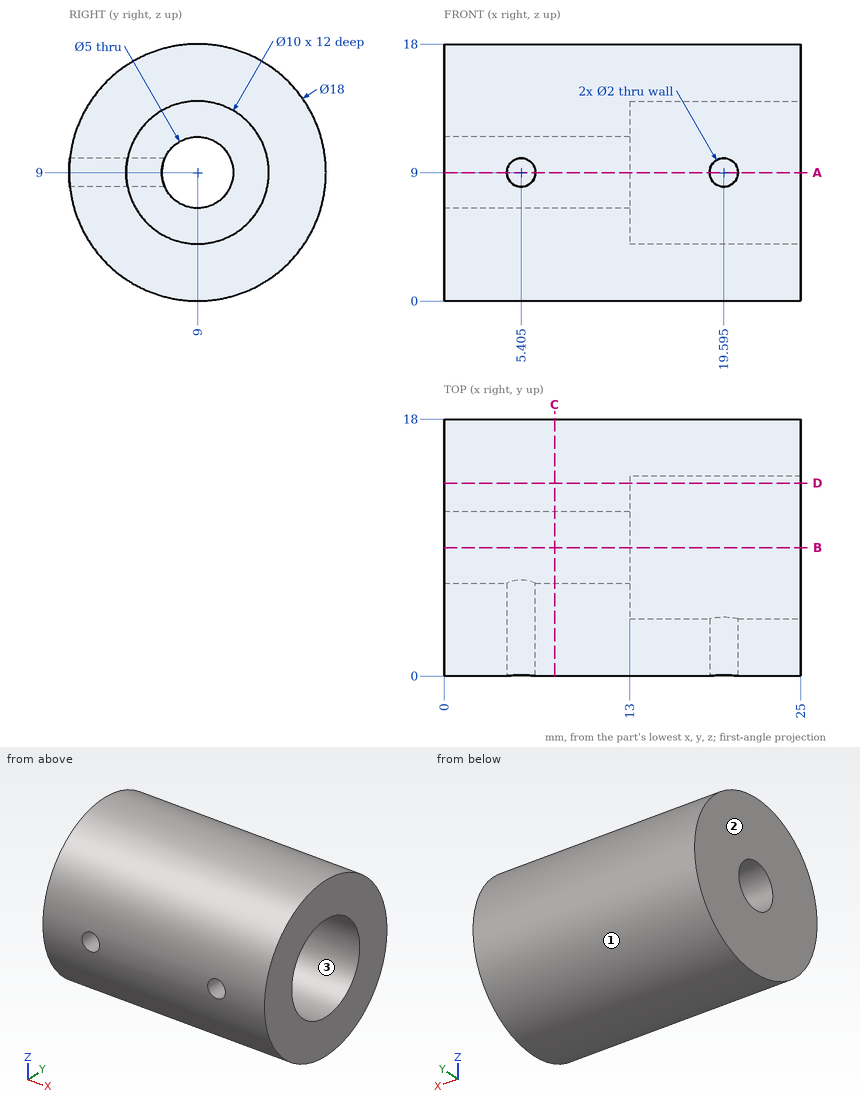
Design review of the part shown in the three views and the two pictorial views. Dimensions are in mm from the part's minimum x, y and z. Coordinates: 2 decimals unless noted, no trailing zeros. Write each loop counter-clockwise with the first axis right and the second up, starting at its lowest first coordinate (ties: lowest second). Pieces come first, ordered by that corner, then holes.
1) We need section A-A on z = 9. State the section outline as (x, y) points (1 decimal).
2) Clearance check with flat-ended pins moving along their axes: pin 1 Ø2 at (x, z) = (6.5, 14.5) entering from -Y (1 decimal); pin 2 Ø1.5 at (x, z) = (19.5, 7) entering from +Y; pin 3 Ø4 at (x, y) = (17.5, 13) entering from +Z (1 decimal). State where each tip first meets the part, or that it passes through.
3) We need section D-D on y = 13.5. State the section outline as (x, z) points (1 decimal), then the cut area to 3 significant figures.
4) We need section B-B on y = 9. State the section outline as (x, z) points.
5) We need section C-C on x = 7.75. State the section outline as (y, z) points.
6) The part is to be moulded in two halves that separate along Z. For the marked faces 1, 2 and 3, say which applies: pulls with the +Z half, pulls with the -Z half, needs draft (parallel to the pull), parting line crosses it, or undercut.
7) To check wall thickness, follow probe 1 along Z at (x, y) = (16.5, 12.25); probe 2 along Z at (x, y) = (22.5, 9); probe 3 along Y at (x, z) = (3.75, 7.5) (1 decimal). State the ranges of each line that lie inside material, in increasing order.
Answer list:
1. outline: (0, 0) - (4.4, 0) - (4.4, 6.5) - (0, 6.5) - close; (0, 11.5) - (13, 11.5) - (13, 14) - (25, 14) - (25, 18) - (0, 18) - close; (6.4, 0) - (18.6, 0) - (18.6, 4) - (13, 4) - (13, 6.5) - (6.4, 6.5) - close; (20.6, 0) - (25, 0) - (25, 4) - (20.6, 4) - close
2. pin 1: stops at y = 1.2
2. pin 2: stops at y = 17.91
2. pin 3: stops at z = 17.8
3. outline: (0, 1.2) - (25, 1.2) - (25, 6.8) - (13, 6.8) - (13, 11.2) - (25, 11.2) - (25, 16.8) - (0, 16.8) - close
3. area: 337 mm2
4. outline: (0, 0) - (25, 0) - (25, 4) - (13, 4) - (13, 6.5) - (0, 6.5) - close; (0, 11.5) - (13, 11.5) - (13, 14) - (25, 14) - (25, 18) - (0, 18) - close
5. outline: circle Ø18 at (9, 9); hole circle Ø5 at (9, 9)
6. face 1: parting line crosses it
6. face 2: needs draft
6. face 3: undercut
7. probe 1: z = 0.61 to 5.2, 12.8 to 17.39
7. probe 2: z = 0 to 4, 14 to 18
7. probe 3: y = 0.1 to 7, 11 to 17.9
